```python
from build123d import *

# Parameters (mm, degrees)
F0_R     = 11.2522
F2_DEPTH = 6.35
F3_DEPTH = 6.35


with BuildPart() as f2:
    # F0 (on Top) → F2 (new body)
    with BuildSketch(Plane.XY):
        with BuildLine():
            ThreePointArc((-11.690817, 65.090521), (-22.647912, 23.556909), (-52.894301, -6.94317))
            ThreePointArc((-52.894301, -6.94317), (-68.099635, -29.944072), (-40.980367, -34.922929))
            ThreePointArc((-40.980367, -34.922929), (-1.688841, -25.706561), (36.828944, -37.754204))
            ThreePointArc((36.828944, -37.754204), (65.008077, -43.265125), (60.898233, -14.847824))
            ThreePointArc((60.898233, -14.847824), (31.044284, 17.814443), (22.80546, 61.290916))
            ThreePointArc((22.80546, 61.290916), (7.677868, 82.442972), (-11.690817, 65.090521))
        make_face()
        with Locations((-52.894301, -23.469558)):
            Circle(F0_R, mode=Mode.SUBTRACT)
        Circle(F0_R, mode=Mode.SUBTRACT)
        with Locations((52.873283, -30.514273)):
            Circle(F0_R, mode=Mode.SUBTRACT)
        with Locations((5.766576, 65.090521)):
            Circle(F0_R, mode=Mode.SUBTRACT)
    extrude(amount=F2_DEPTH)

    # F0 (on Top) → F3 (join)
    with BuildSketch(Plane.XY):
        with BuildLine():
            ThreePointArc((-11.690817, 65.090521), (-22.647912, 23.556909), (-52.894301, -6.94317))
            ThreePointArc((-52.894301, -6.94317), (-68.099635, -29.944072), (-40.980367, -34.922929))
            ThreePointArc((-40.980367, -34.922929), (-1.688841, -25.706561), (36.828944, -37.754204))
            ThreePointArc((36.828944, -37.754204), (65.008077, -43.265125), (60.898233, -14.847824))
            ThreePointArc((60.898233, -14.847824), (31.044284, 17.814443), (22.80546, 61.290916))
            ThreePointArc((22.80546, 61.290916), (7.677868, 82.442972), (-11.690817, 65.090521))
        make_face()
        with Locations((-52.894301, -23.469558)):
            Circle(F0_R, mode=Mode.SUBTRACT)
        Circle(F0_R, mode=Mode.SUBTRACT)
        with Locations((52.873283, -30.514273)):
            Circle(F0_R, mode=Mode.SUBTRACT)
        with Locations((5.766576, 65.090521)):
            Circle(F0_R, mode=Mode.SUBTRACT)
    extrude(amount=F3_DEPTH)


solid = f2.part
```
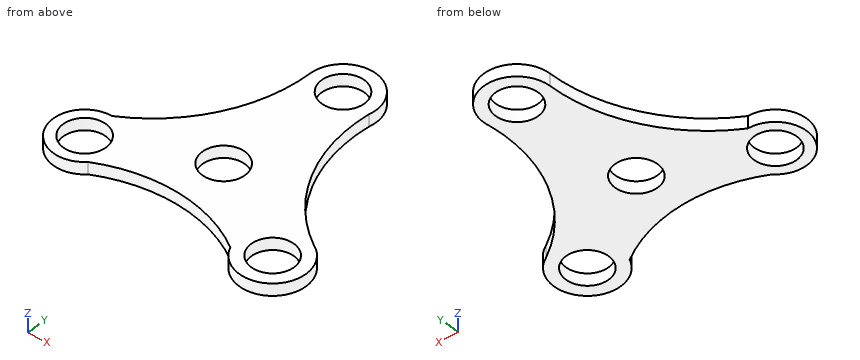
Here's how the part is built. I have some questions about the finished solid (model axes, mm). Round coordinates to 2 decimals unless told otherwise and drop trailing zeros. Order: outer loops, then holes, each group sorted by start corner. A loop starts at its lowest first (then second) coordinate and runs counter-clockwise, first axis right, second up. Notation, with made-up numbers: M 30.25,46 L 48.25,46 A25 cw 48.25,64 Z; hole C 80.5,-5.75 d4. An arc over 180 degrees is marked long. One line per question, with ' | ' between items.
1) I want a section at D-D, the plane y = 20. Write out the boundary of the cut face in (x, z), then the cut area to 3 significant figures.
Working result:
outline: M -24.8,0 L 29.99,0 L 29.99,6.35 L -24.8,6.35 Z | area: 348 mm²
2) I need wall thicknesses on line 1 along X through (y, z) = (64.5, 0.5); line 2 along Y through (x, z) = (0, 4.25); line 3 along Y through (x, z) = (-4, 5.5). Which ranges of each line are inside material? Lowest first, please.
Working result:
line 1: -11.69 to -5.47, 17 to 23.21 | line 2: -25.79 to -11.25, 11.25 to 55.43, 74.75 to 81.57 | line 3: -25.66 to -10.52, 10.52 to 59.5, 70.68 to 79.56
3) For pin 1 Ø1.5 at (x, z) = (-0.5, 2) entering from +Y; pin 2 Ø1 at (y, z) = (-34.5, 3.5) entering from -X, each with a flat end and sliding along its axis, tell me the tip position at first contact or that it passes through.
Working result:
pin 1: y = 81.65 | pin 2: x = -65.63
4) I want a section at A-A, the plane x = 0. Write out the boundary of the cut face in (y, z), then the cut area to 3 significant figures.
Working result:
outline: M -25.79,0 L -11.25,0 L -11.25,6.35 L -25.79,6.35 Z; M 11.25,0 L 55.43,0 L 55.43,6.35 L 11.25,6.35 Z; M 74.75,0 L 81.57,0 L 81.57,6.35 L 74.75,6.35 Z | area: 416 mm²
5) I want a section at B-B, the plane y = 0. Write out the boundary of the cut face in (x, z), then the cut area to 3 significant figures.
Working result:
outline: M -42.79,0 L -11.25,0 L -11.25,6.35 L -42.79,6.35 Z; M 11.25,0 L 43.16,0 L 43.16,6.35 L 11.25,6.35 Z | area: 403 mm²
6) I want a section at C-C, the plane z = 4. Write out the boundary of the cut face in (x, y), then the cut area to 3 significant figures.
Working result:
outline: M -52.89,-6.94 A16.53 ccw long -40.98,-34.92 A76.55 cw 36.83,-37.75 A17.6 ccw long 60.9,-14.85 A81.01 cw 22.81,61.29 A17.46 ccw long -11.69,65.09 A83.03 cw Z; hole C -52.89,-23.47 d22.5; hole C 0,0 d22.5; hole C 5.77,65.09 d22.5; hole C 52.87,-30.51 d22.5 | area: 6,370 mm²
